Read the model definition and answer for the solid it produces. Units are mm, in the model's axes. A direction names the side the tool comes from. Round coordinates to 2 decimals unless told otherwise and drop trailing zeros. Loops run counter-clockwise (first coordinate to the right, second up) from the corner with the lowest first, then second, coordinate; pieces in that order, holes last. Notation, with made-up numbers: M 48.5,27 L 105.5,27 A11 ccw 105.5,39 Z; hole C 41.25,44 d3. An arc over 180 degrees is marked long. Write each question's results on one line, items separated by ' | '.
from build123d import *

# Parameters (mm, degrees)
F0_W     = 12.7
F0_H     = 4.3434
F1_DEPTH = 4.3434
F2_W     = 4.3434
F2_H     = 12.7
F3_DEPTH = 4.3444
F4_R     = 28.880577
F5_DEPTH = 4.3444
F7_DEPTH = 4.3444


with BuildPart() as f1:
    # F0 (on Front) → F1 (new body)
    with BuildSketch(Plane.XZ):
        Polygon((50.8, 74.088349), (0, 100.27007), (-50.8, 74.088349), (-62.088889, 68.270189), (-101.6, 47.906629), (-101.6, -79.093371), (-57.15, -79.093371), (-57.15, -74.749971), (-44.45, -74.749971), (-44.45, -79.093371), (44.45, -79.093371), (44.45, -74.749971), (57.15, -74.749971), (57.15, -79.093371), (101.6, -79.093371), (101.6, 47.906629), (62.088889, 68.270189), align=None)
        Polygon((-62.088889, 68.270189), (-50.8, 74.088349), (-52.789811, 77.949149), (-64.0787, 72.130989), align=None)
        Polygon((52.789811, 77.949149), (50.8, 74.088349), (62.088889, 68.270189), (64.0787, 72.130989), align=None)
        with Locations((-50.8, -76.921671)):
            Rectangle(F0_W, F0_H)
        Polygon((50.8, -79.093371), (57.15, -79.093371), (57.15, -74.749971), (44.45, -74.749971), (44.45, -79.093371), align=None)
    extrude(amount=-F1_DEPTH)

    # F2 (on Front) → F3 (cut, through all)
    with BuildSketch(Plane.XZ):
        with Locations((-99.660009, 0.220258)):
            Rectangle(F2_W, F2_H)
        with Locations((99.660009, 0.220258)):
            Rectangle(F2_W, F2_H)
    extrude(amount=-F3_DEPTH, mode=Mode.SUBTRACT)

    # F4 (on Front) → F5 (cut, through all)
    with BuildSketch(Plane.XZ):
        with Locations((0, 23.649074)):
            Circle(F4_R)
    extrude(amount=-F5_DEPTH, mode=Mode.SUBTRACT)

    # F6 (on Front) → F7 (cut, through all)
    with BuildSketch(Plane.XZ):
        Polygon((-57.15, -79.316832), (-50.8, -79.316832), (-44.45, -79.316832), (-44.45, -74.973432), (-50.8, -74.973432), (-57.15, -74.973432), align=None)
        Polygon((57.15, -79.316832), (57.15, -74.973432), (50.8, -74.973432), (44.45, -74.973432), (44.45, -79.316832), (50.8, -79.316832), align=None)
    extrude(amount=-F7_DEPTH, mode=Mode.SUBTRACT)


solid = f1.part
Item 1: The mould has two halves that part along X. Classify faces 1 (the face through (-80, 2, -79.093)), 2 (the face through (-58.36, 2.14, 75.08)), 3 (the face through (44.45, 2, -77)): pulls with the +X half, pulls with the -X half, needs draft (parallel to the pull), parting line crosses it, or undercut.
Outcome:
face 1: needs draft | face 2: pulls with the -X half | face 3: undercut
Item 2: Straight lines are drawn through the part: line 1 (Z direction, x = 0, y = 2.95); line 2 (Z direction, x = -4, y = 2.3); line 3 (X direction, y = 4.1, z = 73). For each, find the intervals that lie inside material, in ascending order.
Outcome:
line 1: z = -79.09 to -5.23, 52.53 to 100.27 | line 2: z = -79.09 to -4.95, 52.25 to 98.21 | line 3: x = -62.39 to 62.39
Item 3: Flat-ended cylindrical pins translate along their axes: pin 1 (2 mm diameter, centred on y = 1.5, z = -0.5, fed in from -X); pin 2 (2 mm diameter, centred on x = 99, y = 2, fed in from +Z); pin 3 (2 mm diameter, centred on x = -50.5, y = 3, fed in from -Z). Find the tip coordinate at first contact, or state that the pin passes through.
Outcome:
pin 1: stops at x = -97.49 | pin 2: stops at z = 49.76 | pin 3: stops at z = -74.97
Item 4: For faces 4 (the face through (-100, 2, 6.57)), 5 (the face through (-1, 0, -8)), 6 (the face through (57.15, 2, -77)), determine the directions among +Z, -Z, +X, -X, +Y, -Y from which every point of the face is accessible in a straight line to the end or side of a thin tool.
Outcome:
face 4: -X, +Y, -Y | face 5: +Z, -Z, +X, -X, -Y | face 6: -Z, +Y, -Y
Item 5: The part is cut by section A-A (x = -14). Determine the outline of the cut face in (y, z).
Outcome:
outline: M 0,-79.09 L 4.34,-79.09 L 4.34,-1.61 L 0,-1.61 Z; M 0,48.91 L 4.34,48.91 L 4.34,93.05 L 0,93.05 Z
Item 6: The part is cut by section D-D (x = 82). Determine the outline of the cut face in (y, z).
Outcome:
outline: M 0,-79.09 L 4.34,-79.09 L 4.34,58.01 L 0,58.01 Z
Item 7: The part is cut by section B-B (z = 12.5). Determine the outline of the cut face in (x, y), plus the area to 3 significant figures.
Outcome:
outline: M -101.6,0 L -26.64,0 L -26.64,4.34 L -101.6,4.34 Z; M 26.64,0 L 101.6,0 L 101.6,4.34 L 26.64,4.34 Z | area: 651 mm2
